```python
from build123d import *

# Parameters (mm, degrees)
EXTRUDE_1_DEPTH     = 20
SKETCH_2_R          = 21
EXTRUDE_2_DEPTH     = 38
SKETCH_3_R          = 12.5
EXTRUDE_3_DEPTH     = 2
SKETCH_4_R          = 4
EXTRUDE_4_DEPTH     = 18.5
SKETCH_5_R          = 1.75
CUT_EXTRUDE_1_DEPTH = 22.5
SKETCH_6_W          = 5
SKETCH_6_H          = 5
CUT_EXTRUDE_2_DEPTH = 8
CHAMFER_1_SIZE      = 1
SKETCH_7_R          = 12
CUT_EXTRUDE_3_DEPTH = 23
EXTRUDE_5_DEPTH     = 20
SKETCH_9_R          = 2
CUT_EXTRUDE_4_DEPTH = 13


with BuildPart() as part:
    # 草图1 → 凸台-拉伸1 (new body)
    with BuildSketch(Plane(origin=(0, 0, 0), x_dir=(1, 0, 0), z_dir=(0, 1, 0))):
        with BuildLine():
            Line((16.56992758, 21), (-16.56992758, 21))
            ThreePointArc((-16.56992758, 21), (-18.915106397, 18.915106397), (-21, 16.56992758))
            Line((-21, 16.56992758), (-21, -16.56992758))
            ThreePointArc((-21, -16.56992758), (-18.915106397, -18.915106397), (-16.56992758, -21))
            Line((-16.56992758, -21), (16.56992758, -21))
            ThreePointArc((16.56992758, -21), (18.915106397, -18.915106397), (21, -16.56992758))
            Line((21, -16.56992758), (21, 16.56992758))
            ThreePointArc((21, 16.56992758), (18.915106397, 18.915106397), (16.56992758, 21))
        make_face()
    extrude(amount=EXTRUDE_1_DEPTH)

    # 草图2 → 凸台-拉伸2 (add)
    with BuildSketch(Plane(origin=(0, 20, 0), x_dir=(1, 0, 0), z_dir=(0, 1, 0))):
        with Locations(Location((0, 0, 0), (0, 0, 270))):
            Circle(SKETCH_2_R)
    extrude(amount=EXTRUDE_2_DEPTH)

    # 草图3 → 凸台-拉伸3 (add)
    with BuildSketch(Plane(origin=(0, 58, 0), x_dir=(1, 0, 0), z_dir=(0, 1, 0))):
        with Locations(Location((0, 0, 0), (0, 0, 270))):
            Circle(SKETCH_3_R)
    extrude(amount=EXTRUDE_3_DEPTH)

    # 草图4 → 凸台-拉伸4 (add)
    with BuildSketch(Plane(origin=(0, 60, 0), x_dir=(1, 0, 0), z_dir=(0, 1, 0))):
        with Locations(Location((0, 0, 0), (0, 0, 270))):
            Circle(SKETCH_4_R)
    extrude(amount=EXTRUDE_4_DEPTH)

    # 草图5 → 切除-拉伸1 (cut)
    with BuildSketch(Plane.XZ):
        with Locations(Location((15.5, 15.5, 0), (0, 0, 270))):
            Circle(SKETCH_5_R)
        with Locations(Location((15.5, -15.5, 0), (0, 0, 270))):
            Circle(SKETCH_5_R)
        with Locations(Location((-15.5, -15.5, 0), (0, 0, 270))):
            Circle(SKETCH_5_R)
        with Locations(Location((-15.5, 15.5, 0), (0, 0, 270))):
            Circle(SKETCH_5_R)
    extrude(amount=-CUT_EXTRUDE_1_DEPTH, mode=Mode.SUBTRACT)

    # 草图6 → 切除-拉伸2 (cut)
    with BuildSketch(Plane(origin=(0, 20, 0), x_dir=(1, 0, 0), z_dir=(0, 1, 0))):
        with Locations((-15.5, -15.5)):
            Rectangle(SKETCH_6_W, SKETCH_6_H)
        with Locations((15.5, -15.5)):
            Rectangle(SKETCH_6_W, SKETCH_6_H)
        with Locations((-15.5, 15.5)):
            Rectangle(SKETCH_6_W, SKETCH_6_H)
        with Locations((15.5, 15.5)):
            Rectangle(SKETCH_6_W, SKETCH_6_H)
    extrude(amount=CUT_EXTRUDE_2_DEPTH, mode=Mode.SUBTRACT)

    # 倒角1
    chamfer_1_edges = [part.edges().sort_by_distance(p)[0] for p in [
        (13, 24, -13),
        (-13, 24, -13),
        (-13, 24, 13),
        (13, 24, 13),
    ]]
    chamfer(chamfer_1_edges, length=CHAMFER_1_SIZE)

    # 草图7 → 切除-拉伸3 (cut)
    with BuildSketch(Plane.XZ):
        with Locations(Location((0, 0, 0), (0, 0, 270))):
            Circle(SKETCH_7_R)
    extrude(amount=-CUT_EXTRUDE_3_DEPTH, mode=Mode.SUBTRACT)

    # 草图8 → 凸台-拉伸5 (add)
    with BuildSketch(Plane.XZ.offset(-23)):
        with BuildLine():
            ThreePointArc((2.55, 0), (-1.616709621, -1.971991379), (-0.5, 2.50049995))
            Line((-0.5, 2.50049995), (-0.5, 10.988630488))
            ThreePointArc((-0.5, 10.988630488), (-7.599342077, -7.95298686), (11, 0))
            ThreePointArc((11, 0), (7.95298686, 7.599342077), (0.5, 10.988630488))
            Line((0.5, 10.988630488), (0.5, 2.50049995))
            ThreePointArc((0.5, 2.50049995), (1.971991379, 1.616709621), (2.55, 0))
        make_face()
    extrude(amount=EXTRUDE_5_DEPTH)

    # 草图9 → 切除-拉伸4 (cut)
    with BuildSketch(Plane(origin=(0, 58, 0), x_dir=(1, 0, 0), z_dir=(0, 1, 0))):
        with Locations(Location((12.5, 12.5, 0), (0, 0, 270))):
            Circle(SKETCH_9_R)
        with Locations(Location((12.5, -12.5, 0), (0, 0, 270))):
            Circle(SKETCH_9_R)
        with Locations(Location((-12.5, -12.5, 0), (0, 0, 270))):
            Circle(SKETCH_9_R)
        with Locations(Location((-12.5, 12.5, 0), (0, 0, 270))):
            Circle(SKETCH_9_R)
    extrude(amount=-CUT_EXTRUDE_4_DEPTH, mode=Mode.SUBTRACT)


solid = part.part
```
Here's how the part is built. I have some questions about the finished solid (model axes, mm). A direction names the side the tool comes from. Round coordinates to 2 decimals unless told otherwise and drop trailing zeros. Loops run counter-clockwise (first coordinate to the right, second up) from the corner with the lowest first, then second, coordinate; pieces in that order, holes last. Notation, with made-up numbers: (68, -34) -> (115, -34) arc R9 ccw to (115, -28) -> close; hole circle Ø2 at (18, -20.75). An arc over 180 degrees is marked (long way). Answer as CSV lines item,"result". Start each with the question number.
1. For faces 5 (the face through (15, 24, 13)), 6 (the face through (-11.148, 51.591, 11.026)), 7 (the face through (-14, 28, 14)), 8 (the face through (15, 24, -13)), 9 (the face through (-0.5, 13, 7)), which set-ups out of +Z, -Z, +X, -X, +Y, -Y let a thin tool reach every point of the face, with its end or its side?
2. Imagine slicing it at D-D on z = -9. Write out the boundary of the cut face in (x, y), plus the area to 3 significant figures.
3. If we mould it in two halves opening along Z, with no side actions, what happens to faces 1 (the face through (18.88, 9.86, 18.95)), 2 (the face through (17.235, 9.86, -15.272)), 3 (the face through (-8.04, 38.73, 19.4)), 4 (the face through (-13, 24, -15))? For each: pulls with the +Z half, pulls with the -Z half, needs draft (parallel to the pull), parting line crosses it, or undercut.
4. I need wall thicknesses on probe 1 along X at (y, z) = (15.25, 15.5); probe 2 along Z at (x, y) = (-1.5, 9); probe 3 along Z at (x, y) = (15, 7). Which ranges of each line are inside material? Lowest first, please. Write a range as from..to.
5. Imagine slicing it at B-B on x = 15.5. Write out the boundary of the cut face in (y, z), plus the area to 3 significant figures.
6. Imagine slicing it at A-A on y = 47. Write out the boundary of the cut face in (x, z), plus the area to 3 significant figures.
7. I'm going to push flat-ended pins straight in: P1, Ø4, axis at x = -3, z = 14.5, coming from the +Y side; P2, Ø1.7, axis at x = 15, z = -15.5, coming from the -Y side; P3, Ø5, axis at x = 6, y = 45.5, coming from the +Z side. Where does each tip first touch, or does it pass through?
8. Imagine slicing it at C-C on z = 15.5. Write out the boundary of the cut face in (x, y), plus the area to 3 significant figures.
Solution:
1,face 5,"+Z, +X"
1,face 6,"+Y"
1,face 7,"+Z, -X"
1,face 8,"-Z, +X"
1,face 9,"-Y"
2,outline,"(-21, 0) -> (-7.94, 0) -> (-7.94, 23) -> (-6.32, 23) -> (-6.32, 3) -> (6.32, 3) -> (6.32, 23) -> (7.94, 23) -> (7.94, 0) -> (21, 0) -> (21, 20) -> (18.97, 20) -> (18.97, 58) -> (8.67, 58) -> (8.67, 60) -> (-8.67, 60) -> (-8.67, 58) -> (-18.97, 58) -> (-18.97, 20) -> (-21, 20) -> close"
2,area,"2,200 mm²"
3,face 1,"pulls with the +Z half"
3,face 2,"undercut"
3,face 3,"parting line crosses it"
3,face 4,"needs draft"
4,probe 1,"-21..-17.25, -13.75..13.75, 17.25..21"
4,probe 2,"-21..-11.91, -10.9..-2.06, 2.06..10.9, 11.91..21"
4,probe 3,"-21..-17.18, -13.82..13.82, 17.18..21"
5,outline,"(0, -21) -> (20, -21) -> (20, -17.25) -> (0, -17.25) -> close; (0, -13.75) -> (20, -13.75) -> (20, -13) -> (28, -13) -> (28, -14.17) -> (58, -14.17) -> (58, 14.17) -> (28, 14.17) -> (28, 13) -> (20, 13) -> (20, 13.75) -> (0, 13.75) -> close; (0, 17.25) -> (20, 17.25) -> (20, 21) -> (0, 21) -> close"
5,area,"1,760 mm²"
6,outline,"circle Ø42 at (0, 0); hole circle Ø4 at (-12.5, -12.5); hole circle Ø4 at (-12.5, 12.5); hole circle Ø4 at (12.5, -12.5); hole circle Ø4 at (12.5, 12.5)"
6,area,"1,340 mm²"
7,P1,"y = 58"
7,P2,"y = 28"
7,P3,"z = 20.71"
8,outline,"(-21, 0) -> (-17.25, 0) -> (-17.25, 20) -> (-21, 20) -> close; (-14.17, 28) -> (-13, 28) -> (-13, 20) -> (-13.75, 20) -> (-13.75, 0) -> (13.75, 0) -> (13.75, 20) -> (13, 20) -> (13, 28) -> (14.17, 28) -> (14.17, 58) -> (-14.17, 58) -> close; (17.25, 0) -> (21, 0) -> (21, 20) -> (17.25, 20) -> close"
8,area,"1,760 mm²"
